Autodesk Inventor part; units mm, degrees
ref_plane "YZ Plane" through (0, 0, 0) normal (1, 0, 0) x (0, 1, 0)
ref_plane "XZ Plane" through (0, 0, 0) normal (0, 1, 0) x (-1, 0, 0)
ref_plane "XY Plane" through (0, 0, 0) normal (0, 0, 1) x (1, 0, 0)
sketch "Эскиз1" plane through (0, 0, 0) normal (0, 0, 1) x (1, 0, 0)
  line L0 (-41.9106, 11.3854) -> (9.5324, 11.3854)
  line L1 (9.5324, 11.3854) -> (9.5324, -4.2346)
  line L2 (9.5324, -4.2346) -> (-41.9106, -4.2346)
  line L3 (-41.9106, -4.2346) -> (-41.9106, 11.3854)
  point P0 (0, 0)
  dimension "d0" = 51.443
  dimension "d1" = 15.62
extrude "Выдавливание1" add sketch "Эскиз1" against normal blind 16.769
sketch "Эскиз2" plane through (9.5324, -4.2346, 0) normal (1, 0, 0) x (0, 0, -1)
  line L0 (0, 15.62) -> (16.769, 15.62)
  line L1 (16.769, 15.62) -> (-19.74, 15.62)
  line L2 (-19.74, 15.62) -> (-19.74, 0)
  line L3 (-19.74, 0) -> (16.769, 0)
  line L4 (16.769, 0) -> (16.769, 15.62)
  point P0 (0, 4.2346)
  dimension "d4" = 36.509
extrude "Выдавливание2" add sketch "Эскиз2" against normal blind 10
sketch "Эскиз3" plane through (9.5324, -4.2346, -16.769) normal (1, 0, 0) x (0, 0, -1)
  line L0 (0, 15.62) -> (0, 0)
  line L1 (-36.509, 0) -> (0, 0)
  line L2 (-16.769, 0) -> (-21.568, 0)
  line L3 (-21.568, 0) -> (-21.568, 4.078)
  line L4 (-21.568, 4.078) -> (-16.769, 4.078)
  line L5 (-16.769, 4.078) -> (-16.769, 0)
  point P0 (-16.769, 4.2346)
  dimension "d7" = 16.769
  dimension "d8" = 4.799
  dimension "d9" = 4.078
extrude "Выдавливание3" cut sketch "Эскиз3" against normal blind 1.867
sketch "Эскиз4" plane through (-0.4676, -4.2346, 0) normal (-1, 0, 0) x (0, 0, 1)
  line L0 (19.74, 15.62) -> (19.74, 0)
  line L1 (18.24, 1.5) -> (1.5, 1.5)
  line L2 (1.5, 1.5) -> (1.5, 14.12)
  line L3 (1.5, 14.12) -> (18.24, 14.12)
  line L4 (18.24, 14.12) -> (18.24, 1.5)
  point P0 (0, 4.2346)
extrude "Выдавливание4" cut sketch "Эскиз4" against normal blind 7.5
sketch "Эскиз6" plane through (9.5324, -4.2346, -16.769) normal (1, 0, 0) x (0, 0, -1)
  line L0 (-16.769, 0) -> (-36.509, 0)
  line L1 (-21.817, 0) -> (-22.817, 0)
  line L2 (-33.817, 5) -> (-22.817, 5)
  line L3 (-28.317, 6.7654) -> (-28.317, -1.5681)
  line L4 (-36.509, 0) -> (-21.568, 0)
  line L5 (-33.817, 5) -> (-33.817, 0)
  line L6 (-22.817, 5) -> (-22.817, 0)
  line L7 (-35.1049, 6.5) -> (-35.1049, 0)
  line L8 (-35.1049, 0) -> (-33.817, 0)
  line L9 (-35.1049, 6.5) -> (-21.568, 6.5)
  line L10 (-21.568, 6.5) -> (-21.568, 0)
  line L11 (-21.568, 0) -> (-21.568, 4.078)
  line L12 (-21.568, 0) -> (-22.817, 0)
  point P0 (-16.769, 4.2346)
  dimension "d20" = 1
  dimension "d27" = 5
extrude "Выдавливание6" add sketch "Эскиз6" along normal blind 3.817 contours L0 L6 L2 L3 L9 L10 | L3 L2 L5 L0 L7 L9
sketch "Эскиз7" plane through (9.5324, -0.1566, 4.799) normal (0, 0, -1) x (-1, 0, 0)
  line L0 (-3.817, 1.491) -> (0, 2.422)
  line L1 (0, 11.542) -> (0, -4.078)
  line L2 (0, 2.422) -> (-3.817, 2.422)
  line L3 (0, 2.422) -> (-3.817, 2.422)
  line L4 (-3.817, 2.422) -> (-3.817, 1.491)
  point P0 (9.5324, 0.1566)
  point P1 (-3.817, -4.078)
extrude "Выдавливание7" cut sketch "Эскиз7" against normal blind 13.54
sketch "Эскиз8" plane through (-41.9106, -4.2346, -16.769) normal (0, -1, 0) x (1, 0, 0)
  line L0 (51.443, 33.817) -> (55.26, 33.817)
  line L1 (55.26, 33.817) -> (50.26, 33.817)
  line L2 (55.26, 33.817) -> (55.26, 22.817)
  line L3 (55.26, 22.817) -> (50.26, 22.817)
  line L4 (50.26, 22.817) -> (50.26, 33.817)
  line L5 (55.26, 22.817) -> (55.26, 33.817)
  point P0 (41.9106, 16.769)
  dimension "d33" = 5
  dimension "d34" = 5
extrude "Выдавливание8" cut sketch "Эскиз8" against normal blind 5
sketch "Эскиз10" plane through (8.3494, -4.2346, 17.048) normal (1, 0, 0) x (0, 0, -1)
  line L0 (0, 0) -> (0, 5)
  line L1 (0, 5) -> (0, 1)
  line L2 (0, 1) -> (11, 1)
  line L3 (11, 5) -> (11, 0)
  line L4 (11, 1) -> (11, 5)
  line L5 (0, 5) -> (11, 5)
  line L6 (11, 5) -> (0, 5)
  point P0 (17.048, 4.2346)
  dimension "d38" = 4
extrude "Выдавливание9" cut sketch "Эскиз10" against normal blind 10
sketch "Эскиз11" plane through (-0.4676, -4.2346, 0) normal (-1, 0, 0) x (0, 0, 1)
  line L0 (17.048, 0) -> (17.048, 5)
  line L1 (18.3359, 5.569) -> (18.3359, 0)
  line L2 (18.3359, 0.9988) -> (18.3359, 14.12)
  line L3 (1.5, 14.12) -> (18.24, 14.12)
  line L4 (18.3359, 14.12) -> (1.5, 14.12)
  line L5 (1.5, 14.12) -> (1.5, 0.9988)
  line L6 (1.5, 1.5) -> (1.5, 14.12)
  line L7 (1.5, 0.9988) -> (18.3359, 0.9988)
  point P0 (0, 4.2346)
extrude "Выдавливание10" cut sketch "Эскиз11" against normal blind 7.817
properties part number "Батарейка"
Could you check a few things on this model? Use its own coordinates, in mm. A direction names the side the tool comes from. Round coordinates to 2 decimals unless told otherwise and drop trailing zeros. Loops run counter-clockwise (first coordinate to the right, second up) from the corner with the lowest first, then second, coordinate; pieces in that order, holes last. Notation, with made-up numbers: M 5,17 L 56,17 A29 cw 56,50 Z; hole C -24.75,81 d2. An arc over 180 degrees is marked long. Put each result on its own line as item: value.
Q1. Imagine slicing it at C-C (y = 7). Write out the boundary of the cut face in (x, z).
Check result:
outline: M -41.91,-16.77 L 9.53,-16.77 L 9.53,19.74 L -0.47,19.74 L -0.47,18.34 L 7.35,18.34 L 7.35,1.5 L -0.47,1.5 L -0.47,0 L -41.91,0 Z
Q2. Imagine slicing it at D-D (x = -23). Write out the boundary of the cut face in (y, z).
Check result:
outline: M -4.23,-16.77 L 11.39,-16.77 L 11.39,0 L -4.23,0 Z
Q3. On a 3-axis mill with a long thin cutter (end or side, diameter ignored), from which of +Z, -Z, +X, -X, +Y, -Y can I reach the whole of each face in a straight line? I mean faces 1 (the face through (9, -2, 0)), 2 (the face through (5, 4, 19.74)), 3 (the face through (3, -3.236, 10)), 4 (the face through (-21, 4, 0)), 5 (the face through (11, -1, 18.336)). Say none if no direction works.
Check result:
face 1: +X, -Y
face 2: +Z, +X, -X, +Y, -Y
face 3: -X
face 4: +Z, -X, +Y, -Y
face 5: +Z, +X, +Y, -Y
Q4. I need wall thicknesses on probe 1 along Z at (x, y) = (4, 1.25); probe 2 along Y at (x, z) = (8, 14); probe 3 along X at (y, z) = (5.5, -2.5). Which ranges of each line are inside material? Lowest first, please.
Check result:
probe 1: -16.77 to 1.5, 18.34 to 19.74
probe 2: -4.23 to -3.23, 0.77 to 11.39
probe 3: -41.91 to 9.53
Q5. For pin 1 (1.1 mm diameter, centred on x = 11, y = 0.5, fed in from +Z); pin 2 (1.5 mm diameter, centred on x = 8.5, z = 1.5, fed in from -Y); pin 3 (8 mm diameter, centred on y = 2.5, z = 10.5, fed in from -X), each with a flat end and sliding along its axis, tell me the tip position at first contact or that it passes through.
Check result:
pin 1: z = 18.34
pin 2: y = -0.16
pin 3: x = 7.35
Q6. Imagine slicing it at B-B (y = -1.25). Write out the boundary of the cut face in (x, z), then the cut area to 3 significant figures.
Check result:
outline: M -41.91,-16.77 L 9.53,-16.77 L 9.53,0 L 7.67,0 L 7.67,4.8 L 13.35,4.8 L 13.35,6.05 L 7.35,6.05 L 7.35,1.5 L -0.47,1.5 L -0.47,0 L -41.91,0 Z; M -0.47,18.34 L 7.35,18.34 L 7.35,17.05 L 13.35,17.05 L 13.35,18.34 L 9.53,18.34 L 9.53,19.74 L -0.47,19.74 Z
area: 905 mm2
Q7. Thinking about a two-plate mould opening in Y: for faces 6 (the face through (3, 3, 18.336)), 7 (the face through (-11, 11.385, -6)), 8 (the face through (-0.468, 11, 10)), which applies, released by +Y, released by -Y, zero draft, split by the parting line, or undercut?
Check result:
face 6: undercut
face 7: released by +Y
face 8: zero draft
